```python
from build123d import *

# Parameters (mm, degrees)
SKETCH1_W           = 164.1
SKETCH1_H           = 174.745
SKETCH1_R           = 1.5875
SKETCH1_R_2         = 14.462
BOSS_EXTRUDE1_DEPTH = 1.5875
FILLET1_R           = 1


with BuildPart() as part:
    # Sketch1 → Boss-Extrude1 (new body)
    with BuildSketch(Plane.XY):
        with Locations((82.55, -87.3725)):
            Rectangle(SKETCH1_W, SKETCH1_H)
        with BuildLine():
            Line((16.934372699, -168.395), (19.05, -168.395))
            ThreePointArc((19.05, -168.395), (20.6375, -169.9825), (19.05, -171.57))
            Line((19.05, -171.57), (16.934372699, -171.57))
            ThreePointArc((16.934372699, -171.57), (12.1625, -169.9825), (16.934372699, -168.395))
        make_face(mode=Mode.SUBTRACT)
        with BuildLine():
            Line((7.409372699, -151.9325), (9.525, -151.9325))
            ThreePointArc((9.525, -151.9325), (11.1125, -153.52), (9.525, -155.1075))
            Line((9.525, -155.1075), (7.409372699, -155.1075))
            ThreePointArc((7.409372699, -155.1075), (2.6375, -153.52), (7.409372699, -151.9325))
        make_face(mode=Mode.SUBTRACT)
        with BuildLine():
            Line((42.334372699, -168.395), (44.45, -168.395))
            ThreePointArc((44.45, -168.395), (46.0375, -169.9825), (44.45, -171.57))
            Line((44.45, -171.57), (42.334372699, -171.57))
            ThreePointArc((42.334372699, -171.57), (37.5625, -169.9825), (42.334372699, -168.395))
        make_face(mode=Mode.SUBTRACT)
        with BuildLine():
            Line((67.734372699, -168.395), (69.85, -168.395))
            ThreePointArc((69.85, -168.395), (71.4375, -169.9825), (69.85, -171.57))
            Line((69.85, -171.57), (67.734372699, -171.57))
            ThreePointArc((67.734372699, -171.57), (62.9625, -169.9825), (67.734372699, -168.395))
        make_face(mode=Mode.SUBTRACT)
        with BuildLine():
            Line((7.409372699, -126.5325), (9.525, -126.5325))
            ThreePointArc((9.525, -126.5325), (11.1125, -128.12), (9.525, -129.7075))
            Line((9.525, -129.7075), (7.409372699, -129.7075))
            ThreePointArc((7.409372699, -129.7075), (2.6375, -128.12), (7.409372699, -126.5325))
        make_face(mode=Mode.SUBTRACT)
        with BuildLine():
            Line((7.409372699, -101.1325), (9.525, -101.1325))
            ThreePointArc((9.525, -101.1325), (11.1125, -102.72), (9.525, -104.3075))
            Line((9.525, -104.3075), (7.409372699, -104.3075))
            ThreePointArc((7.409372699, -104.3075), (2.6375, -102.72), (7.409372699, -101.1325))
        make_face(mode=Mode.SUBTRACT)
        with BuildLine():
            Line((93.134372699, -168.395), (95.25, -168.395))
            ThreePointArc((95.25, -168.395), (96.8375, -169.9825), (95.25, -171.57))
            Line((95.25, -171.57), (93.134372699, -171.57))
            ThreePointArc((93.134372699, -171.57), (88.3625, -169.9825), (93.134372699, -168.395))
        make_face(mode=Mode.SUBTRACT)
        with BuildLine():
            Line((118.534372699, -168.395), (120.65, -168.395))
            ThreePointArc((120.65, -168.395), (122.2375, -169.9825), (120.65, -171.57))
            Line((120.65, -171.57), (118.534372699, -171.57))
            ThreePointArc((118.534372699, -171.57), (113.7625, -169.9825), (118.534372699, -168.395))
        make_face(mode=Mode.SUBTRACT)
        with BuildLine():
            Line((143.934372699, -168.395), (146.05, -168.395))
            ThreePointArc((146.05, -168.395), (147.6375, -169.9825), (146.05, -171.57))
            Line((146.05, -171.57), (143.934372699, -171.57))
            ThreePointArc((143.934372699, -171.57), (139.1625, -169.9825), (143.934372699, -168.395))
        make_face(mode=Mode.SUBTRACT)
        with BuildLine():
            Line((159.809372699, -151.9325), (161.925, -151.9325))
            ThreePointArc((161.925, -151.9325), (163.5125, -153.52), (161.925, -155.1075))
            Line((161.925, -155.1075), (159.809372699, -155.1075))
            ThreePointArc((159.809372699, -155.1075), (155.0375, -153.52), (159.809372699, -151.9325))
        make_face(mode=Mode.SUBTRACT)
        with Locations((82.55, -100.966)):
            Circle(SKETCH1_R, mode=Mode.SUBTRACT)
        with BuildLine():
            Line((159.809372699, -126.5325), (161.925, -126.5325))
            ThreePointArc((161.925, -126.5325), (163.5125, -128.12), (161.925, -129.7075))
            Line((161.925, -129.7075), (159.809372699, -129.7075))
            ThreePointArc((159.809372699, -129.7075), (155.0375, -128.12), (159.809372699, -126.5325))
        make_face(mode=Mode.SUBTRACT)
        with BuildLine():
            Line((159.809372699, -101.1325), (161.925, -101.1325))
            ThreePointArc((161.925, -101.1325), (163.5125, -102.72), (161.925, -104.3075))
            Line((161.925, -104.3075), (159.809372699, -104.3075))
            ThreePointArc((159.809372699, -104.3075), (155.0375, -102.72), (159.809372699, -101.1325))
        make_face(mode=Mode.SUBTRACT)
        with BuildLine():
            Line((7.409372699, -75.7325), (9.525, -75.7325))
            ThreePointArc((9.525, -75.7325), (11.1125, -77.32), (9.525, -78.9075))
            Line((9.525, -78.9075), (7.409372699, -78.9075))
            ThreePointArc((7.409372699, -78.9075), (2.6375, -77.32), (7.409372699, -75.7325))
        make_face(mode=Mode.SUBTRACT)
        with BuildLine():
            Line((7.409372699, -50.3325), (9.525, -50.3325))
            ThreePointArc((9.525, -50.3325), (11.1125, -51.92), (9.525, -53.5075))
            Line((9.525, -53.5075), (7.409372699, -53.5075))
            ThreePointArc((7.409372699, -53.5075), (2.6375, -51.92), (7.409372699, -50.3325))
        make_face(mode=Mode.SUBTRACT)
        with Locations((65.659, -84.075)):
            Circle(SKETCH1_R, mode=Mode.SUBTRACT)
        with BuildLine():
            Line((7.409372699, -24.9325), (9.525, -24.9325))
            ThreePointArc((9.525, -24.9325), (11.1125, -26.52), (9.525, -28.1075))
            Line((9.525, -28.1075), (7.409372699, -28.1075))
            ThreePointArc((7.409372699, -28.1075), (2.6375, -26.52), (7.409372699, -24.9325))
        make_face(mode=Mode.SUBTRACT)
        with BuildLine():
            Line((7.409372699, -8.1), (9.525, -8.1))
            ThreePointArc((9.525, -8.1), (11.1125, -9.6875), (9.525, -11.275))
            Line((9.525, -11.275), (7.409372699, -11.275))
            ThreePointArc((7.409372699, -11.275), (2.6375, -9.6875), (7.409372699, -8.1))
        make_face(mode=Mode.SUBTRACT)
        with BuildLine():
            Line((29.634372699, -2.2625), (31.75, -2.2625))
            ThreePointArc((31.75, -2.2625), (33.3375, -3.85), (31.75, -5.4375))
            Line((31.75, -5.4375), (29.634372699, -5.4375))
            ThreePointArc((29.634372699, -5.4375), (24.8625, -3.85), (29.634372699, -2.2625))
        make_face(mode=Mode.SUBTRACT)
        with BuildLine():
            Line((55.034372699, -2.2625), (57.15, -2.2625))
            ThreePointArc((57.15, -2.2625), (58.7375, -3.85), (57.15, -5.4375))
            Line((57.15, -5.4375), (55.034372699, -5.4375))
            ThreePointArc((55.034372699, -5.4375), (50.2625, -3.85), (55.034372699, -2.2625))
        make_face(mode=Mode.SUBTRACT)
        with BuildLine():
            Line((80.434372699, -2.2625), (82.55, -2.2625))
            ThreePointArc((82.55, -2.2625), (84.1375, -3.85), (82.55, -5.4375))
            Line((82.55, -5.4375), (80.434372699, -5.4375))
            ThreePointArc((80.434372699, -5.4375), (75.6625, -3.85), (80.434372699, -2.2625))
        make_face(mode=Mode.SUBTRACT)
        with Locations((82.55, -84.075)):
            Circle(SKETCH1_R_2, mode=Mode.SUBTRACT)
        with Locations((99.441, -84.075)):
            Circle(SKETCH1_R, mode=Mode.SUBTRACT)
        with Locations((82.55, -67.184)):
            Circle(SKETCH1_R, mode=Mode.SUBTRACT)
        with BuildLine():
            Line((159.809372699, -75.7325), (161.925, -75.7325))
            ThreePointArc((161.925, -75.7325), (163.5125, -77.32), (161.925, -78.9075))
            Line((161.925, -78.9075), (159.809372699, -78.9075))
            ThreePointArc((159.809372699, -78.9075), (155.0375, -77.32), (159.809372699, -75.7325))
        make_face(mode=Mode.SUBTRACT)
        with BuildLine():
            Line((159.809372699, -50.3325), (161.925, -50.3325))
            ThreePointArc((161.925, -50.3325), (163.5125, -51.92), (161.925, -53.5075))
            Line((161.925, -53.5075), (159.809372699, -53.5075))
            ThreePointArc((159.809372699, -53.5075), (155.0375, -51.92), (159.809372699, -50.3325))
        make_face(mode=Mode.SUBTRACT)
        with BuildLine():
            Line((105.834372699, -2.2625), (107.95, -2.2625))
            ThreePointArc((107.95, -2.2625), (109.5375, -3.85), (107.95, -5.4375))
            Line((107.95, -5.4375), (105.834372699, -5.4375))
            ThreePointArc((105.834372699, -5.4375), (101.0625, -3.85), (105.834372699, -2.2625))
        make_face(mode=Mode.SUBTRACT)
        with BuildLine():
            Line((159.809372699, -24.9325), (161.925, -24.9325))
            ThreePointArc((161.925, -24.9325), (163.5125, -26.52), (161.925, -28.1075))
            Line((161.925, -28.1075), (159.809372699, -28.1075))
            ThreePointArc((159.809372699, -28.1075), (155.0375, -26.52), (159.809372699, -24.9325))
        make_face(mode=Mode.SUBTRACT)
        with BuildLine():
            Line((131.234372699, -2.2625), (133.35, -2.2625))
            ThreePointArc((133.35, -2.2625), (134.9375, -3.85), (133.35, -5.4375))
            Line((133.35, -5.4375), (131.234372699, -5.4375))
            ThreePointArc((131.234372699, -5.4375), (126.4625, -3.85), (131.234372699, -2.2625))
        make_face(mode=Mode.SUBTRACT)
        with BuildLine():
            Line((159.809372699, -8.1), (161.925, -8.1))
            ThreePointArc((161.925, -8.1), (163.5125, -9.6875), (161.925, -11.275))
            Line((161.925, -11.275), (159.809372699, -11.275))
            ThreePointArc((159.809372699, -11.275), (155.0375, -9.6875), (159.809372699, -8.1))
        make_face(mode=Mode.SUBTRACT)
    extrude(amount=BOSS_EXTRUDE1_DEPTH)

    # Fillet1
    fillet1_edges = [part.edges().sort_by_distance(p)[0] for p in [
        (0.5, -174.745, 0.79375),
        (0.5, 0, 0.79375),
        (164.6, 0, 0.79375),
        (164.6, -174.745, 0.79375),
    ]]
    fillet(fillet1_edges, radius=FILLET1_R)


solid = part.part
```
Geometry: final body of the model. Coordinates: model frame, mm. Coordinates: 2 decimals unless noted, no trailing zeros. Return JSON: item names as keys, results as strings. Group by question number.
1. Pull-direction query (X, two-part tool) for faces 1 (the face through (139.164, -170.075, 0.783)), 2 (the face through (2.64, -9.78, 0.78)); classes: pulls with the +X half, pulls with the -X half, needs draft (parallel to the pull), parting line crosses it, or undercut.
2. Pin query (flat end, axial travel): pin 1 (8.5 mm diameter, centred on x = 5.29, y = -153.52, fed in from +Z); pin 2 (3 mm diameter, centred on x = 157.69, y = -102.72, fed in from -Z). Return the tip coordinate at first contact, or that it passes through.
3. Material intervals for line 1 along Y through (x, z) = (142, 0.1) (3 decimals); line 2 along Y through (x, z) = (99.5, 0.75) (3 decimals); line 3 along X through (y, z) = (-153.52, 1.25), sorted ascending. Write a range as [from, to].
4. Cut plane A-A (z = 1.05). Count the separate pieces of the cut face and the enclosed holes in it, plus the area to 3 significant figures.
Resolved:
{
 "1": {"face 1": "undercut", "face 2": "undercut"},
 "2": {"pin 1": "stops at z = 1.59", "pin 2": "passes through"},
 "3": {"line 1": "y = [-174.745, -172.626], [-167.339, 0]", "line 2": "y = [-174.745, -85.661], [-82.489, 0]", "line 3": "x = [0.5, 2.64], [11.11, 155.04], [163.51, 164.6]"},
 "4": {"separate pieces": "1", "enclosed holes": "30", "area": "27,200 mm²"}
}
